For this review, use the dimensioned drawing (mm, ordinates from the lowest corner) and the shaded views. A direction names the side the tool comes from. Round coordinates to 2 decimals unless told otherwise and drop trailing zeros. Order: outer loops, then holes, each group sorted by start corner. A loop starts at its lowest first (then second) coordinate and runs counter-clockwise, first axis right, second up. Notation, with made-up numbers: M 31,20.5 L 87,20.5 A14 ccw 87,37.5 Z; hole C 57.25,23 d10. An arc over 180 degrees is marked long. One line per item, written item: value. Start each with the question number.
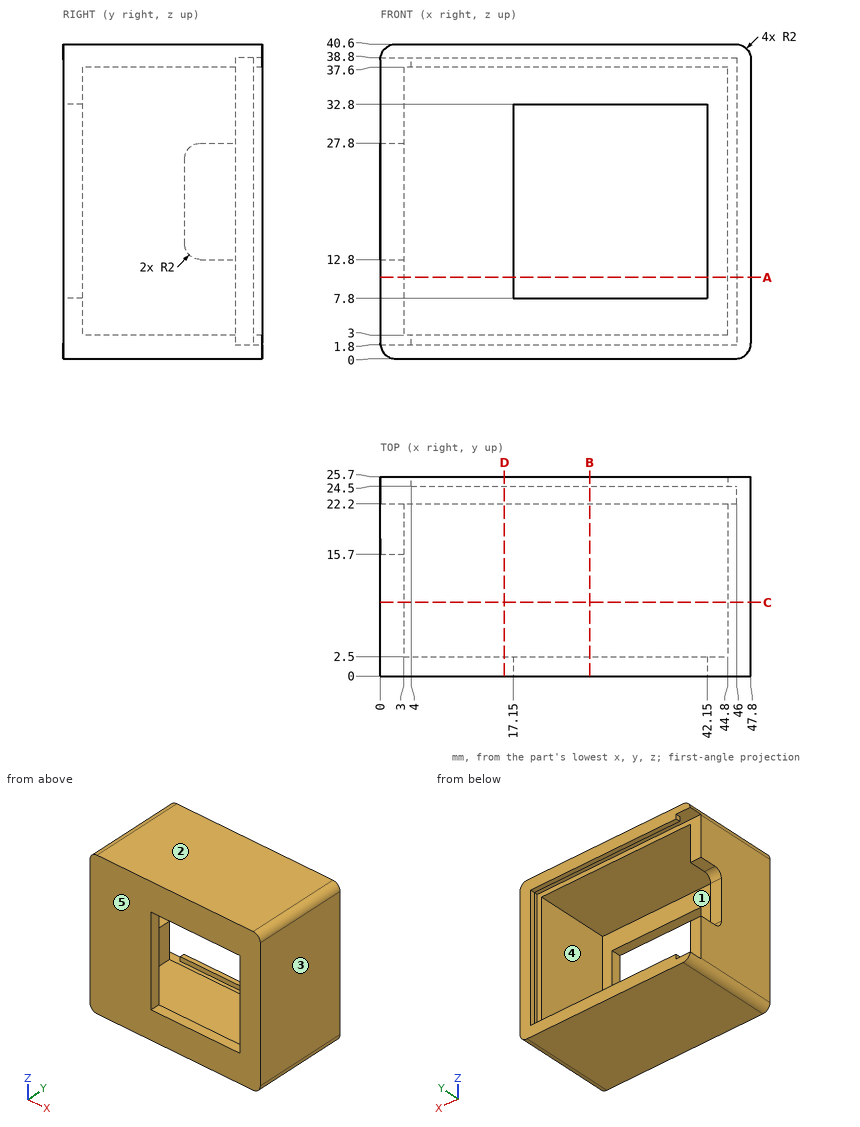
Item 1: Wall thickness on L1, parallel to Z at x = 15, y = 15; L2, parallel to X at y = 15, z = 11; L3, parallel to Y at x = 45, z = 30.5: over which ranges is each line inside the solid? List them lowest first.
Item 2: Consider section B-B, the plane x = 27. Give the boundary of the cut face in (y, z).
Item 3: Consider section D-D, the plane x = 16. Give the boundary of the cut face in (y, z), then the cut area to 3 significant figures.
Item 4: Consider section C-C, the plane y = 9.5. Give the boundary of the cut face in (x, z).
Item 5: Consider section A-A, the plane z = 10.5. Give the boundary of the cut face in (x, y), then the cut area to 3 significant figures.
Item 6: Machinability: for the marked faces 4 and 5, which of the approach directions +Z, -Z, +X, -X, +Y, -Y give a long, thin tool a straight path to every point of the face, cutting with its end or side? Answer none if there is none.
Item 7: Clearance check with flat-ended pins moving along their axes: P1, Ø10.5, axis at x = 18, z = 12.5, coming from the +Y side; P2, Ø1.2, axis at y = 23, z = 21, coming from the -X side; P3, Ø1.3, axis at y = 25, z = 20.5, coming from the -X side. State where each tip first meets the part, or that it passes through.
Item 8: The part is to be moulded in two halves that separate along X. For the marked faces 1, 2 and 3, say which applies: pulls with the +X half, pulls with the -X half, needs draft (parallel to the pull), parting line crosses it, or undercut.
Computed:
1. L1: z = 0 to 3, 37.6 to 40.6
1. L2: x = 0 to 3, 44.8 to 47.8
1. L3: y = 0 to 22.2, 24.5 to 25.7
2. outline: M 0,0 L 25.7,0 L 25.7,3 L 24.5,3 L 24.5,1.8 L 22.2,1.8 L 22.2,3 L 2.5,3 L 2.5,7.8 L 0,7.8 Z; M 0,32.8 L 2.5,32.8 L 2.5,37.6 L 22.2,37.6 L 22.2,38.8 L 24.5,38.8 L 24.5,37.6 L 25.7,37.6 L 25.7,40.6 L 0,40.6 Z
3. outline: M 0,0 L 25.7,0 L 25.7,3 L 24.5,3 L 24.5,1.8 L 22.2,1.8 L 22.2,3 L 2.5,3 L 2.5,37.6 L 22.2,37.6 L 22.2,38.8 L 24.5,38.8 L 24.5,37.6 L 25.7,37.6 L 25.7,40.6 L 0,40.6 Z
3. area: 235 mm^2
4. outline: M 0,2 A2 ccw 2,0 L 45.8,0 A2 ccw 47.8,2 L 47.8,38.6 A2 ccw 45.8,40.6 L 2,40.6 A2 ccw 0,38.6 Z; hole M 3,3 L 44.8,3 L 44.8,37.6 L 3,37.6 Z
5. outline: M 0,0 L 17.15,0 L 17.15,2.5 L 3,2.5 L 3,22.2 L 0,22.2 Z; M 42.15,0 L 47.8,0 L 47.8,25.7 L 44.8,25.7 L 44.8,24.5 L 46,24.5 L 46,22.2 L 44.8,22.2 L 44.8,2.5 L 42.15,2.5 Z
5. area: 183 mm^2
6. face 4: +Y
6. face 5: +Z, -Z, +X, -X, -Y
7. P1: stops at y = 2.5
7. P2: stops at x = 46
7. P3: stops at x = 44.8
8. face 1: undercut
8. face 2: needs draft
8. face 3: pulls with the +X half
